from build123d import *

# Parameters (mm, degrees)
BOSS_EXTRUDE1_DEPTH     = 12.5
BOSS_EXTRUDE2_DEPTH     = 2.5
BOSS_EXTRUDE3_DEPTH     = 2.5
CUT_EXTRUDE1_DEPTH      = 51.023744362
SKETCH5_R               = 2.4
CUT_EXTRUDE2_DEPTH      = 32.5
SKETCH6_R               = 2.4
CUT_EXTRUDE3_DEPTH      = 32.5
CUT_EXTRUDE4_DEPTH      = 12.5
CUT_EXTRUDE4_DEPTH_BACK = 12.5
SKETCH7_R               = 4.25
CUT_EXTRUDE5_DEPTH      = 12.5
CUT_EXTRUDE5_DEPTH_BACK = 12.5
SKETCH8_R               = 4.25


with BuildPart() as part:
    # Sketch1 → Boss-Extrude1 (new body)
    with BuildSketch(Plane(origin=(0, 0, 0), x_dir=(1, 0, 0), z_dir=(0, 1, 0))):
        Polygon((-31.75, 31.75), (31.75, -31.75), (31.75, 31.75), align=None)
    extrude(amount=BOSS_EXTRUDE1_DEPTH)

    # Sketch2 → Boss-Extrude2 (add)
    with BuildSketch(Plane(origin=(31.75, 0, 0), x_dir=(0, 0, -1), z_dir=(1, 0, 0))):
        with BuildLine():
            Line((26.05, 4.4), (27.25, 4.4))
            ThreePointArc((27.25, 4.4), (28.310660172, 4.839339828), (28.75, 5.9))
            Line((28.75, 5.9), (28.75, 7.1))
            ThreePointArc((28.75, 7.1), (28.310660172, 8.160660172), (27.25, 8.6))
            Line((27.25, 8.6), (26.05, 8.6))
            ThreePointArc((26.05, 8.6), (24.989339828, 8.160660172), (24.55, 7.1))
            Line((24.55, 7.1), (24.55, 5.9))
            ThreePointArc((24.55, 5.9), (24.989339828, 4.839339828), (26.05, 4.4))
        make_face()
        with BuildLine():
            Line((11.85, 5.9), (11.85, 7.1))
            ThreePointArc((11.85, 7.1), (12.289339828, 8.160660172), (13.35, 8.6))
            Line((13.35, 8.6), (14.55, 8.6))
            ThreePointArc((14.55, 8.6), (15.610660172, 8.160660172), (16.05, 7.1))
            Line((16.05, 7.1), (16.05, 5.9))
            ThreePointArc((16.05, 5.9), (15.610660172, 4.839339828), (14.55, 4.4))
            Line((14.55, 4.4), (13.35, 4.4))
            ThreePointArc((13.35, 4.4), (12.289339828, 4.839339828), (11.85, 5.9))
        make_face()
        with BuildLine():
            Line((-0.85, 5.9), (-0.85, 7.1))
            ThreePointArc((-0.85, 7.1), (-0.410660172, 8.160660172), (0.65, 8.6))
            Line((0.65, 8.6), (1.85, 8.6))
            ThreePointArc((1.85, 8.6), (2.910660172, 8.160660172), (3.35, 7.1))
            Line((3.35, 7.1), (3.35, 5.9))
            ThreePointArc((3.35, 5.9), (2.910660172, 4.839339828), (1.85, 4.4))
            Line((1.85, 4.4), (0.65, 4.4))
            ThreePointArc((0.65, 4.4), (-0.410660172, 4.839339828), (-0.85, 5.9))
        make_face()
        with BuildLine():
            Line((-13.55, 5.9), (-13.55, 7.1))
            ThreePointArc((-13.55, 7.1), (-13.110660172, 8.160660172), (-12.05, 8.6))
            Line((-12.05, 8.6), (-10.85, 8.6))
            ThreePointArc((-10.85, 8.6), (-9.789339828, 8.160660172), (-9.35, 7.1))
            Line((-9.35, 7.1), (-9.35, 5.9))
            ThreePointArc((-9.35, 5.9), (-9.789339828, 4.839339828), (-10.85, 4.4))
            Line((-10.85, 4.4), (-12.05, 4.4))
            ThreePointArc((-12.05, 4.4), (-13.110660172, 4.839339828), (-13.55, 5.9))
        make_face()
        with BuildLine():
            Line((-26.25, 5.9), (-26.25, 7.1))
            ThreePointArc((-26.25, 7.1), (-25.810660172, 8.160660172), (-24.75, 8.6))
            Line((-24.75, 8.6), (-23.55, 8.6))
            ThreePointArc((-23.55, 8.6), (-22.489339828, 8.160660172), (-22.05, 7.1))
            Line((-22.05, 7.1), (-22.05, 5.9))
            ThreePointArc((-22.05, 5.9), (-22.489339828, 4.839339828), (-23.55, 4.4))
            Line((-23.55, 4.4), (-24.75, 4.4))
            ThreePointArc((-24.75, 4.4), (-25.810660172, 4.839339828), (-26.25, 5.9))
        make_face()
    extrude(amount=BOSS_EXTRUDE2_DEPTH)

    # Sketch3 → Boss-Extrude3 (add)
    with BuildSketch(Plane(origin=(0, 0, -31.75), x_dir=(-1, 0, 0), z_dir=(0, 0, -1))):
        with BuildLine():
            Line((-26.05, 4.4), (-27.25, 4.4))
            ThreePointArc((-27.25, 4.4), (-28.310660172, 4.839339828), (-28.75, 5.9))
            Line((-28.75, 5.9), (-28.75, 7.1))
            ThreePointArc((-28.75, 7.1), (-28.310660172, 8.160660172), (-27.25, 8.6))
            Line((-27.25, 8.6), (-26.05, 8.6))
            ThreePointArc((-26.05, 8.6), (-24.989339828, 8.160660172), (-24.55, 7.1))
            Line((-24.55, 7.1), (-24.55, 5.9))
            ThreePointArc((-24.55, 5.9), (-24.989339828, 4.839339828), (-26.05, 4.4))
        make_face()
        with BuildLine():
            Line((-11.85, 5.9), (-11.85, 7.1))
            ThreePointArc((-11.85, 7.1), (-12.289339828, 8.160660172), (-13.35, 8.6))
            Line((-13.35, 8.6), (-14.55, 8.6))
            ThreePointArc((-14.55, 8.6), (-15.610660172, 8.160660172), (-16.05, 7.1))
            Line((-16.05, 7.1), (-16.05, 5.9))
            ThreePointArc((-16.05, 5.9), (-15.610660172, 4.839339828), (-14.55, 4.4))
            Line((-14.55, 4.4), (-13.35, 4.4))
            ThreePointArc((-13.35, 4.4), (-12.289339828, 4.839339828), (-11.85, 5.9))
        make_face()
        with BuildLine():
            Line((0.85, 5.9), (0.85, 7.1))
            ThreePointArc((0.85, 7.1), (0.410660172, 8.160660172), (-0.65, 8.6))
            Line((-0.65, 8.6), (-1.85, 8.6))
            ThreePointArc((-1.85, 8.6), (-2.910660172, 8.160660172), (-3.35, 7.1))
            Line((-3.35, 7.1), (-3.35, 5.9))
            ThreePointArc((-3.35, 5.9), (-2.910660172, 4.839339828), (-1.85, 4.4))
            Line((-1.85, 4.4), (-0.65, 4.4))
            ThreePointArc((-0.65, 4.4), (0.410660172, 4.839339828), (0.85, 5.9))
        make_face()
        with BuildLine():
            Line((13.55, 5.9), (13.55, 7.1))
            ThreePointArc((13.55, 7.1), (13.110660172, 8.160660172), (12.05, 8.6))
            Line((12.05, 8.6), (10.85, 8.6))
            ThreePointArc((10.85, 8.6), (9.789339828, 8.160660172), (9.35, 7.1))
            Line((9.35, 7.1), (9.35, 5.9))
            ThreePointArc((9.35, 5.9), (9.789339828, 4.839339828), (10.85, 4.4))
            Line((10.85, 4.4), (12.05, 4.4))
            ThreePointArc((12.05, 4.4), (13.110660172, 4.839339828), (13.55, 5.9))
        make_face()
        with BuildLine():
            Line((26.25, 5.9), (26.25, 7.1))
            ThreePointArc((26.25, 7.1), (25.810660172, 8.160660172), (24.75, 8.6))
            Line((24.75, 8.6), (23.55, 8.6))
            ThreePointArc((23.55, 8.6), (22.489339828, 8.160660172), (22.05, 7.1))
            Line((22.05, 7.1), (22.05, 5.9))
            ThreePointArc((22.05, 5.9), (22.489339828, 4.839339828), (23.55, 4.4))
            Line((23.55, 4.4), (24.75, 4.4))
            ThreePointArc((24.75, 4.4), (25.810660172, 4.839339828), (26.25, 5.9))
        make_face()
    extrude(amount=BOSS_EXTRUDE3_DEPTH)

    # Sketch4 → Cut-Extrude1 (cut, through all)
    with BuildSketch(Plane(origin=(0, 12.5, 0), x_dir=(1, 0, 0), z_dir=(0, 1, 0))):
        Polygon((31.75, -2.434304015), (-2.434304015, 31.75), (-2.434304015, 36.268787218), (35.715446441, 36.268787218), (35.715446441, -2.434304015), align=None)
    extrude(amount=-CUT_EXTRUDE1_DEPTH, mode=Mode.SUBTRACT)

    # Sketch5 → Cut-Extrude2 (cut)
    with BuildSketch(Plane(origin=(34.25, 0, 0), x_dir=(0, 0, -1), z_dir=(1, 0, 0))):
        with Locations(Location((-11.45, 6.5, 0), (0, 0, 180))):
            Circle(SKETCH5_R)
    extrude(amount=-CUT_EXTRUDE2_DEPTH, mode=Mode.SUBTRACT)

    # Sketch6 → Cut-Extrude3 (cut)
    with BuildSketch(Plane(origin=(0, 0, -34.25), x_dir=(-1, 0, 0), z_dir=(0, 0, -1))):
        with Locations((11.45, 6.5)):
            Circle(SKETCH6_R)
    extrude(amount=-CUT_EXTRUDE3_DEPTH, mode=Mode.SUBTRACT)

    # Sketch7 → Cut-Extrude4 (cut, two sides: drawn at the far end of the back side and taken through both)
    with BuildSketch(Plane.XY.offset(-9.811165381).offset(-CUT_EXTRUDE4_DEPTH_BACK)):
        with Locations(Location((-11.45, 6.5, 0), (0, 0, 180))):
            Circle(SKETCH7_R)
    extrude(amount=CUT_EXTRUDE4_DEPTH + CUT_EXTRUDE4_DEPTH_BACK, mode=Mode.SUBTRACT)

    # Sketch8 → Cut-Extrude5 (cut, two sides: drawn at the far end of the back side and taken through both)
    with BuildSketch(Plane.ZY.offset(-10.09384537).offset(-CUT_EXTRUDE5_DEPTH_BACK)):
        with Locations((11.45, 6.5)):
            Circle(SKETCH8_R)
    extrude(amount=CUT_EXTRUDE5_DEPTH + CUT_EXTRUDE5_DEPTH_BACK, mode=Mode.SUBTRACT)


solid = part.part
Read the model definition and answer for the solid it produces. Units are mm, in the model's axes. A direction names the side the tool comes from. Coordinates: 2 decimals unless noted, no trailing zeros. Loops run counter-clockwise (first coordinate to the right, second up) from the corner with the lowest first, then second, coordinate; pieces in that order, holes last. Notation, with made-up numbers: (10.25, 8) - (61.25, 8) arc R4 cw to (61.25, 14) - close; hole circle Ø8 at (-18, 77). An arc over 180 degrees is marked (long way). Answer in a Markdown table with one row per item.
Q1. For faces 1 (the cylindrical face through (-7.204, 6.313, -16.473)), 2 (the cylindrical face through (32.98, 8.15, 25.82)), 3 (the flat face through (22.594, 4.7, 13.3)), 4 (the cylindrical face through (32.98, 8.17, 22.5)), determine the directions among +Z, -Z, +X, -X, +Y, -Y from which every point of the face is accessible in a straight line to the end or side of a thin tool.
Here are the results:
| item | result |
|---|---|
| face 1 | +Z |
| face 2 | +Z, +X, +Y |
| face 3 | -X |
| face 4 | -Z, +X, +Y |
Q2. Find section D-D on z = -5. Write down the section's boundary in (x, y), plus the area to 3 significant figures.
Here are the results:
| item | result |
|---|---|
| outline | (-5, 0) - (24.32, 0) - (24.32, 12.5) - (-5, 12.5) - close |
| area | 366 mm^2 |
Q3. The mould has two halves that part along Z. Classify faces 5 (the cylindrical face through (16.648, 6.687, 7.204)), 6 (the flat face through (0, 6, 0)), 7 (the cylindrical face through (-25.8, 4.83, -32.98)): pulls with the +Z half, pulls with the -Z half, needs draft (parallel to the pull), parting line crosses it, or undercut.
Here are the results:
| item | result |
|---|---|
| face 5 | undercut |
| face 6 | pulls with the +Z half |
| face 7 | needs draft |
Q4. Straight lines are drawn through the part: line 1 along Y through (x, z) = (25.25, 11.45); line 2 along Y through (x, z) = (16.25, 11.45); line 3 along X through (y, z) = (6.75, -29.5). For each, find the intervals that lie inside material, in ascending order. Write a range as [from, to].
Here are the results:
| item | result |
|---|---|
| line 1 | y = [0, 4.1], [8.9, 12.5] |
| line 2 | y = [0, 2.25], [10.75, 12.5] |
| line 3 | x = [-29.5, -13.84], [-9.06, -0.18] |
Q5. Find section A-A on x = -11.45. Write down the section's boundary in (y, z), plus the area to 3 significant figures.
Here are the results:
| item | result |
|---|---|
| outline | (0, -31.75) - (4.1, -31.75) - (4.1, -22.31) - (2.25, -22.31) - (2.25, -11.45) - (0, -11.45) - close; (8.9, -31.75) - (12.5, -31.75) - (12.5, -11.45) - (10.75, -11.45) - (10.75, -22.31) - (8.9, -22.31) - close |
| area | 116 mm^2 |
Q6. Find section C-C on z = -23.5. Write down the section's boundary in (x, y).
Here are the results:
| item | result |
|---|---|
| outline | (-23.5, 0) - (5.82, 0) - (5.82, 12.5) - (-23.5, 12.5) - close; hole circle Ø4.8 at (-11.45, 6.5) |
Q7. Find section B-B on z = 11.45. Write down the section's boundary in (x, y).
Here are the results:
| item | result |
|---|---|
| outline | (11.45, 0) - (31.75, 0) - (31.75, 4.1) - (22.59, 4.1) - (22.59, 2.25) - (11.45, 2.25) - close; (11.45, 10.75) - (22.59, 10.75) - (22.59, 8.9) - (31.75, 8.9) - (31.75, 12.5) - (11.45, 12.5) - close |
Q8. Given P1, Ø1, axis at x = 32.5, z = 24, coming from the -Y side; P2, Ø1, axis at x = -24, z = -33.5, coming from the +Y side; P3, Ø6, axis at y = 6.5, z = 11.45, coming from the -X side; P4, Ø6, axis at y = 9, z = 21.5, coming from the +X side, each flat-ended and moving along its own axis, determine where each tip first touches the part or whether it passes through.
Here are the results:
| item | result |
|---|---|
| P1 | stops at y = 4.4 |
| P2 | stops at y = 8.6 |
| P3 | stops at x = 22.59 |
| P4 | stops at x = 34.25 |
